Job drawing, mm, ordinate dimensions from the low corner. One solid piece. Coordinates: 2 decimals unless noted, no trailing zeros. Write each loop counter-clockwise with the first axis right and the second up, starting at its lowest first coordinate (ties: lowest second). Pieces come first, ordered by that corner, then holes. Notation, with made-up numbers: (25.5, 77) - (54.5, 77) arc R19 cw to (54.5, 87) - close; hole circle Ø1 at (32.5, 21.5). An arc over 180 degrees is marked (long way). Use a Markdown table: item, result.
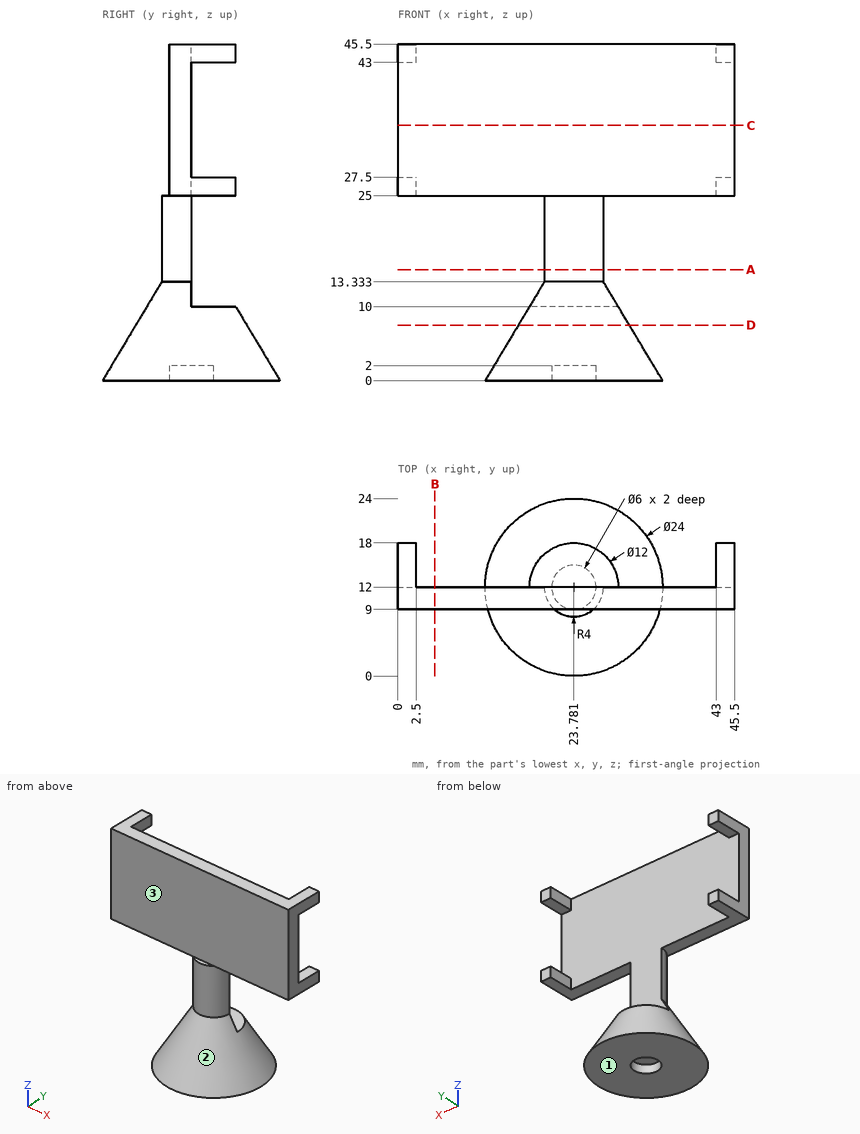
Item 1: Band-saw the part on B-B, the plane x = 5. Give the cut face in (y, z).
From the geometry:
| item | result |
|---|---|
| outline | (9, 25) - (12, 25) - (12, 45.5) - (9, 45.5) - close |
Item 2: Band-saw the part on C-C, the plane z = 34.5. Give the cut face in (x, y).
From the geometry:
| item | result |
|---|---|
| outline | (0, 9) - (45.5, 9) - (45.5, 12) - (0, 12) - close |
Item 3: Drop flat-ended pins along their axis: P1, Ø3, axis at x = 23.5, y = 11.5, coming from the -Z side; P2, Ø2.5, axis at x = 35.5, y = 14.5, coming from the -Z side; P3, Ø10, axis at x = 27.5, z = 31.5, coming from the -Y side; P4, Ø2, axis at x = 1, z = 44.5, coming from the +Y side. Give the stop position or say it passes through.
From the geometry:
| item | result |
|---|---|
| P1 | z = 2 |
| P2 | z = 0 |
| P3 | y = 9 |
| P4 | y = 18 |
Item 4: Drill centre lines: probe 1 along Y at (x, z) = (34.5, 33); probe 2 along Z at (x, y) = (20, 9.5) (1 decimal); probe 3 along Z at (x, y) = (26.5, 16.5). Where is each one in solid material? Low to high.
From the geometry:
| item | result |
|---|---|
| probe 1 | 9 to 12 |
| probe 2 | 0 to 12.4, 25 to 45.5 |
| probe 3 | 0 to 10 |
Item 5: Two-plate mould, pull along Z, no slides. Class the marked faces 1, 2 and 3: pulls with the +Z half, pulls with the -Z half, needs draft (parallel to the pull), parting line crosses it, or undercut.
From the geometry:
| item | result |
|---|---|
| face 1 | pulls with the -Z half |
| face 2 | undercut |
| face 3 | needs draft |
Item 6: Band-saw the part on A-A, the plane z = 15. Give the cut face in (x, y), then the cut area to 3 significant figures.
From the geometry:
| item | result |
|---|---|
| outline | (19.78, 12) arc R4 ccw to (27.78, 12) - close |
| area | 25.1 mm^2 |
Item 7: Band-saw the part on D-D, the plane z = 7.5. Give the cut face in (x, y), then the cut area to 3 significant figures.
From the geometry:
| item | result |
|---|---|
| outline | circle Ø15 at (23.78, 12) |
| area | 177 mm^2 |
